The model under review builds one solid part; all positions refer to its coordinate system, in mm. Face numbers are marked on the shaded views. A direction names the side the tool comes from. Coordinates: 2 decimals unless noted, no trailing zeros. Order: outer loops, then holes, each group sorted by start corner. A loop starts at its lowest first (then second) coordinate and runs counter-clockwise, first axis right, second up. Notation, with made-up numbers: M 62,-24.5 L 112,-24.5 A25 ccw 112,2.5 Z; hole C 27,54 d7. An arc over 180 degrees is marked long. Answer as CSV lines item,"result". Start each with the question number.
Q1. Wall thickness on L1, parallel to Z at x = 0, y = -3.5; L2, parallel to X at y = -9.9, z = 0; L3, parallel to Y at x = -2.25, z = 2 (3 decimals): over which ranges is each line inside the solid? List them lowest first. Write a range as [from, to].
Q2. Machinability: for the marked faces 1, 2 and 3, which of the approach directions +Z, -Z, +X, -X, +Y, -Y give a long, thin tool a straight path to every point of the face, cutting with its end or side? Answer none if there is none.
Q3. Consider section B-B on y = -4.75. Write out the cut boundary in (x, z).
Q4. For P1, Ø2, axis at x = 0, z = 0, coming from the -Y side, flat-tipped, find the tip position at first contact; note if it passes through.
Q5. Consider section A-A on x = 0.75. Write out the cut boundary in (y, z) (3 decimals), and give its area (3 significant figures).
Q6. Consider section C-C on z = 2.25. Write out the cut boundary in (x, y) (3 decimals).
Q7. The part is to be moulded in two halves that separate along Z. For the marked faces 4 and 5, say which applies: +Z half, -Z half, draft (parallel to the pull), parting line (faces both ways), or undercut.
Q8. Consider section D-D on x = -3.5. Write out the cut boundary in (y, z) (3 decimals).
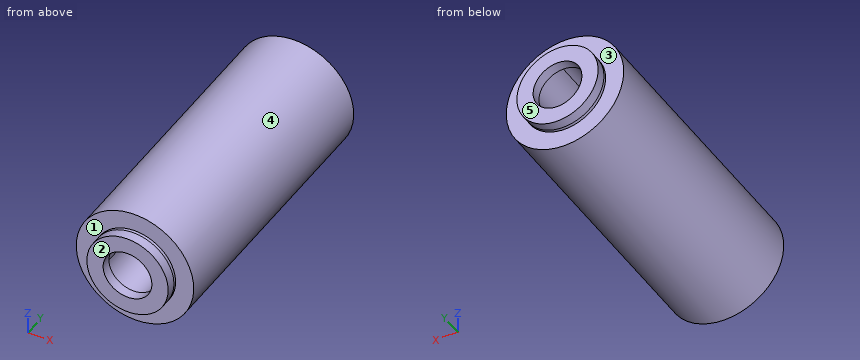
from build123d import *

# Parameters (mm, degrees)
SKETCH2_R                = 3.9751
BOSS_EXTRUDE1_DEPTH      = 9.525
M4X0_7_TAPPED_HOLE1_D    = 3.3
SKETCH5_R                = 2.75
SKETCH5_R_2              = 1.65
BOSS_EXTRUDE2_DEPTH      = 0.675
BOSS_EXTRUDE2_DEPTH_BACK = 19.725
SKETCH6_R                = 3.9751
SKETCH6_R_2              = 2.75
CUT_EXTRUDE1_DEPTH       = 0.2
SKETCH7_R                = 3.9751
SKETCH7_R_2              = 2.75
CUT_EXTRUDE2_DEPTH       = 0.2


with BuildPart() as part:
    # Sketch2 → Boss-Extrude1 (new, symmetric)
    with BuildSketch(Plane(origin=(0, 0, 0), x_dir=(1, 0, 0), z_dir=(0, 1, 0))):
        with Locations(Location((0, 0, 0), (0, 0, 90))):
            Circle(SKETCH2_R)
    extrude(amount=BOSS_EXTRUDE1_DEPTH, both=True)

    # M4x0.7 Tapped Hole1 (through all)
    with Locations(Plane(origin=(0, 9.525, 0), x_dir=(1, 0, 0), z_dir=(0, 1, 0))):
        with Locations((0, 0)):
            Hole(M4X0_7_TAPPED_HOLE1_D / 2)

    # Sketch5 → Boss-Extrude2 (add, two sides)
    with BuildSketch(Plane(origin=(0, 9.525, 0), x_dir=(1, 0, 0), z_dir=(0, 1, 0))) as boss_extrude2_sk:
        with Locations(Location((0, 0, 0), (0, 0, 270))):
            Circle(SKETCH5_R)
        with Locations(Location((0, 0, 0), (0, 0, 270))):
            Circle(SKETCH5_R_2, mode=Mode.SUBTRACT)
    extrude(amount=BOSS_EXTRUDE2_DEPTH)
    extrude(boss_extrude2_sk.sketch, amount=-BOSS_EXTRUDE2_DEPTH_BACK)

    # Sketch6 → Cut-Extrude1 (cut)
    with BuildSketch(Plane(origin=(0, 9.525, 0), x_dir=(1, 0, 0), z_dir=(0, 1, 0))):
        with Locations(Location((0, 0, 0), (0, 0, 90))):
            Circle(SKETCH6_R)
        with Locations(Location((0, 0, 0), (0, 0, 270))):
            Circle(SKETCH6_R_2, mode=Mode.SUBTRACT)
    extrude(amount=-CUT_EXTRUDE1_DEPTH, mode=Mode.SUBTRACT)

    # Sketch7 → Cut-Extrude2 (cut)
    with BuildSketch(Plane.XZ.offset(9.525)):
        with Locations(Location((0, 0, 0), (0, 0, 270))):
            Circle(SKETCH7_R)
        with Locations(Location((0, 0, 0), (0, 0, 90))):
            Circle(SKETCH7_R_2, mode=Mode.SUBTRACT)
    extrude(amount=-CUT_EXTRUDE2_DEPTH, mode=Mode.SUBTRACT)


solid = part.part
Evaluation:
1,L1,"z = [-3.98, -1.65], [1.65, 3.98]"
1,L2,"x = [-2.75, -1.65], [1.65, 2.75]"
1,L3,"y = [-9.325, 9.325]"
2,face 1,"-Y"
2,face 2,"+Z, -Z, +X, -X, -Y"
2,face 3,"+Y"
3,outline,"C 0,0 d7.95; hole C 0,0 d3.3"
4,P1,"passes through"
5,outline,"M -10.2,-2.646 L -9.325,-2.646 L -9.325,-3.904 L 9.325,-3.904 L 9.325,-2.646 L 10.2,-2.646 L 10.2,-1.47 L -10.2,-1.47 Z; M -10.2,1.47 L 10.2,1.47 L 10.2,2.646 L 9.325,2.646 L 9.325,3.904 L -9.325,3.904 L -9.325,2.646 L -10.2,2.646 Z"
5,area,"94.9 mm²"
6,outline,"M -3.277,-9.325 L -1.581,-9.325 L -1.581,-10.2 L 1.581,-10.2 L 1.581,-9.325 L 3.277,-9.325 L 3.277,9.325 L 1.581,9.325 L 1.581,10.2 L -1.581,10.2 L -1.581,9.325 L -3.277,9.325 Z"
7,face 4,"parting line"
7,face 5,"draft"
8,outline,"M -9.325,-1.885 L 9.325,-1.885 L 9.325,1.885 L -9.325,1.885 Z"
